Autodesk Inventor part; units mm, degrees
ref_plane "YZ Plane" through (0, 0, 0) normal (1, 0, 0) x (0, 1, 0)
ref_plane "XZ Plane" through (0, 0, 0) normal (0, 1, 0) x (-1, 0, 0)
ref_plane "XY Plane" through (0, 0, 0) normal (0, 0, 1) x (1, 0, 0)
sketch "Sketch1" plane through (0, 0, 0) normal (0, 0, 1) x (1, 0, 0)
  line L0 (0, 0) -> (0, 101.6) construction
  line L1 (0, 101.6) -> (30.48, 101.6) construction
  line L2 (30.48, 101.6) -> (30.48, 0)
  arc A0 (30.48, 0) -> (30.48, 101.6) centre (30.48, 50.8) ccw
  line L3 (31.98, 1.5228) -> (31.98, 100.0772)
  arc A1 (31.98, 1.5228) -> (31.98, 100.0772) centre (30.48, 50.8) ccw
  dimension "d0" = 30.48
  dimension "d1" = 101.6
  dimension "d2" = 50.8
  dimension "d3" = 1.5
revolve "Revolution1" add sketch "Sketch1" angle 360 about axis through (0, 0, 0) along (0, 1, 0)
sketch "Sketch2" plane through (0, 0, 0) normal (0, 1, 0) x (-1, 0, 0)
  line L0 (0, 0) -> (-38.1, 0) construction
  circle A0 centre (-38.1, 0) radius 3
  dimension "d5" = 6
  dimension "d6" = 38.1
extrude "Extrusion1" cut sketch "Sketch2" along normal blind 101.6
pattern_circular "Circular Pattern1" count 3 over 360 about axis through (0, 50.8, 0) along (0, 1, 0) of "Extrusion1"
properties part number "Buoy 6 FatHalfSphere_3DPrint"
Design review of the part built by this model. Coordinates are the model's own, in mm. Round coordinates to 2 decimals unless told otherwise and drop trailing zeros. Return JSON: item names as keys, results as strings.
Q1. The part is to be moulded in two halves that separate along Y. For faces 1 (the cylindrical face through (35.24, 100.15, -0.9)), 2 (the cylindrical face through (-6.93, 51.49, 31.22)), say which applies: pulls with the +Y half, pulls with the -Y half, needs draft (parallel to the pull), parting line crosses it, or undercut.
Computed values:
{"face 1": "needs draft", "face 2": "undercut"}
Q2. Consider section A-A on x = 0. Give the number of separate pieces and of enclosed holes in the cut face, plus the area to 3 significant figures.
Computed values:
{"separate pieces": "2", "enclosed holes": "2", "area": "767 mm2"}
Q3. For pin 1 Ø3 at (x, y) = (-20, 26) entering from -Z; pin 2 Ø10 at (x, y) = (29, 50.5) entering from +Z; pin 3 Ø4 at (x, z) = (-12, -41.5) entering from -Y; pin 4 Ø5 at (x, z) = (-19.05, -33) entering from +Y, all flat-tipped, find the tip position at first contact; note any pin that passes through.
Computed values:
{"pin 1": "stops at z = -73.02", "pin 2": "stops at z = 77.66", "pin 3": "stops at y = 1.14", "pin 4": "passes through"}
Q4. Wall thickness on L1, parallel to X at y = 50.5, z = 3; L2, parallel to X at y = 91.5, z = 26; L3, parallel to Z at x = 26, y = 7.5: over which ranges is each line inside the solid? List them lowest first. Write a range as [from, to].
Computed values:
{"L1": "x = [-81.22, -79.72], [-31.84, -30.33], [30.33, 31.84], [79.72, 81.22]", "L2": "x = [-55.05, -52.18], [-18.62, -15.91], [15.91, 18.62], [52.18, 55.05]", "L3": "z = [-50.78, -47.39], [-18.62, -15.91], [15.91, 18.62], [47.39, 50.78]"}
